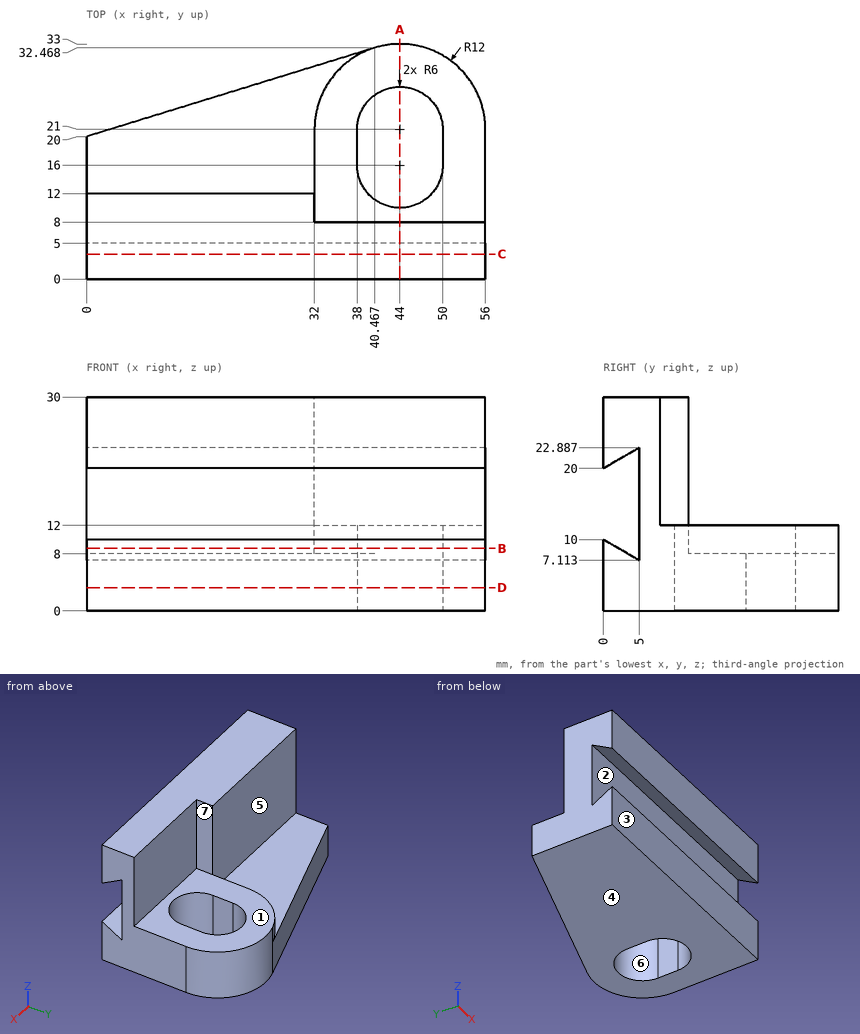
Verification items for this drawing (mm, ordinates from the low corner). A direction names the side the tool comes from. Give positions to 0.01 mm unless a question says otherwise; leave off trailing zeros. Write each loop counter-clockwise with the first axis right and the second up, starting at its lowest first coordinate (ties: lowest second). Pieces come first, ordered by that corner, then holes. Notation, with made-up numbers: (12, -17) - (27, -17) arc R17 cw to (27, -2) - close; hole circle Ø7 at (59, 30.5). An arc over 180 degrees is marked (long way). Answer as a JSON object with one key per item and string values. Group by question number.
1) Sectioned sample at C-C (y = 3.5). Record the cut outline in (x, z).
2) Sectioned sample at D-D (z = 3.25). Record the cut outline in (x, y), then the cut area to 3 significant figures.
3) Thickness scan on probe 1 along X at (y, z) = (16.5, 6); probe 2 along Y at (x, z) = (4, 11.5); probe 3 along Z at (x, y) = (42.5, 28.5). Record the ranges inside material, lowest first. Write a range as from..to.
4) Depth check by flat-ended pin: P1, Ø10, axis at x = 35.5, y = 24, coming from the +Z side; P2, Ø1.2, axis at y = 10.5, z = 23, coming from the +X side; P3, Ø16.5, axis at x = 14.5, y = 20, coming from the +Z side; P4, Ø8, axis at x = 8, z = 15.5, coming from the +Y side. Enter the tip coordinate at first touch or a pass-through.
5) Sectioned sample at B-B (z = 8.75). Record the cut outline in (x, y) (1 decimal).
6) Sectioned sample at A-A (x = 44). Record the cut outline in (y, z).
7) Release check for a two-part mould opening along Y. For the marked faces 1, 2 and 3 record: pulls with the +Y half, pulls with the -Y half, needs draft (parallel to the pull), parting line crosses it, or undercut.
8) Access from +Z, -Z, +X, -X, +Y, -Y to the whole of each face (thin tool, end or side, straight path). Record for the marked faces 4, 5, 6 and 7.
Geometry results:
{
 "1": {"outline": "(0, 0) - (56, 0) - (56, 7.98) - (0, 7.98) - close; (0, 22.02) - (56, 22.02) - (56, 30) - (0, 30) - close"},
 "2": {"outline": "(0, 0) - (56, 0) - (56, 21) arc R12 ccw to (40.47, 32.47) - (0, 20) - close; hole (38, 16) arc R6 ccw to (50, 16) - (50, 21) arc R6 ccw to (38, 21) - close", "area": "1,370 mm^2"},
 "3": {"probe 1": "x = 0..38, 50..56", "probe 2": "y = 5..12", "probe 3": "z = 0..12"},
 "4": {"P1": "stops at z = 12", "P2": "stops at x = 32", "P3": "stops at z = 30", "P4": "stops at y = 12"},
 "5": {"outline": "(0, 0) - (56, 0) - (56, 2.2) - (0, 2.2) - close; (0, 5) - (56, 5) - (56, 21) arc R12 ccw to (32, 21) - (32, 12) - (0, 12) - close; hole (38, 16) arc R6 ccw to (50, 16) - (50, 21) arc R6 ccw to (38, 21) - close"},
 "6": {"outline": "(0, 0) - (10, 0) - (10, 12) - (8, 12) - (8, 30) - (0, 30) - (0, 20) - (5, 22.89) - (5, 7.11) - (0, 10) - close; (27, 0) - (33, 0) - (33, 12) - (27, 12) - close"},
 "7": {"face 1": "needs draft", "face 2": "undercut", "face 3": "pulls with the -Y half"},
 "8": {"face 4": "-Z, +X, -X, +Y, -Y", "face 5": "+Z, -X, +Y", "face 6": "+Z, -Z", "face 7": "+Z, +X, +Y"}
}
